Design review of the part built by this model. Coordinates are the model's own, in mm. Face numbers are marked on the shaded views. A direction names the side the tool comes from. Give positions to 0.01 mm unless a question says otherwise; leave off trailing zeros. Write each loop counter-clockwise with the first axis right and the second up, starting at its lowest first coordinate (ties: lowest second). Pieces come first, ordered by that corner, then holes. Notation, with made-up numbers: (-30, 62) -> (14, 62) arc R15 cw to (14, 80) -> close; hole circle Ø1 at (2.25, 27). An arc over 180 degrees is marked (long way). Return JSON: item names as keys, results as strings. Group by question number.
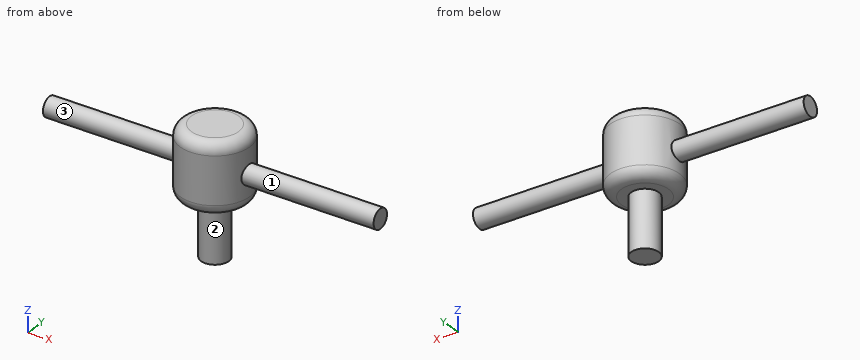
from build123d import *

# Parameters (mm, degrees)
F0_R     = 15.875
F1_DEPTH = 31.75
F2_R     = 4.445
F3_DEPTH = 76.2
F4_R     = 4.445
F5_DEPTH = 76.2
F6_R     = 6.35
F7_DEPTH = 25.908
F8_R     = 5.08


with BuildPart() as f1:
    # F0 (on Top) → F1 (new body)
    with BuildSketch(Plane.XY):
        Circle(F0_R)
    extrude(amount=F1_DEPTH)

    # F2 (on Right) → F3 (join)
    with BuildSketch(Plane.YZ):
        with Locations((0, 14.891451)):
            Circle(F2_R)
    extrude(amount=F3_DEPTH)

    # F4 (on Right) → F5 (join)
    with BuildSketch(Plane.YZ):
        with Locations((0, 14.891451)):
            Circle(F4_R)
    extrude(amount=-F5_DEPTH)

    # F6 (on face) → F7 (join)
    with BuildSketch(Plane(origin=(0, 0, 0), x_dir=(1, 0, 0), z_dir=(0, 0, -1))):
        Circle(F6_R)
    extrude(amount=F7_DEPTH)

    # F8
    f8_edges = [f1.edges().sort_by_distance(p)[0] for p in [
        (-15.875, 0, 31.75),
        (-15.875, 0, 0),
    ]]
    fillet(f8_edges, radius=F8_R)


solid = f1.part
Q1. Insertion check: pin 1 (12 mm diameter, centred on x = 28, z = 6, fed in from +Y); pin 2 (4 mm diameter, centred on y = 11, z = 6, fed in from -X); pin 3 (12 mm diameter, centred on x = -19.5, y = 8, fed in from -Z). Each pin has a flat end and moves straight along its axis. Give the tip position at first contact, or say it passes through.
Q2. Take a section at B-B, the plane x = 0. Give the boundary of the cut face in (y, z) (3 decimals), plus the area to 3 significant figures.
Q3. For L1, parallel to X at y = 4.5, z = 23.5; L2, parallel to Z at x = 62, y = 0.5; L3, parallel to X at y = 8, z = 8.5, list the stretches that pass through material, from the lowest coordinate up. Write a range as from..to.
Q4. Tool access review of the marked faces 1, 2 and 3: name each direction out of +Z, -Z, +X, -X, +Y, -Y from which nothing blocks a thin tool from reaching the whole face with its end or side.
Q5. Take a section at C-C, the plane z = 18. Give the boundary of the cut face in (x, y) (3 decimals), plus the area to 3 significant figures.
Q6. Take a section at A-A, the plane y = 0. Give the boundary of the cut face in (x, z) (3 decimals), plus the area to 3 significant figures.
Q7. Take a section at D-D, the plane z = 6.5. Give the boundary of the cut face in (x, y) (3 decimals), plus the area to 3 significant figures.
Final values:
{
 "1": {"pin 1": "stops at y = 3.38", "pin 2": "stops at x = -13.08", "pin 3": "stops at z = 2.35"},
 "2": {"outline": "(-15.875, 5.08) arc R5.08 ccw to (-10.795, 0) -> (-6.35, 0) -> (-6.35, -25.908) -> (6.35, -25.908) -> (6.35, 0) -> (10.795, 0) arc R5.08 ccw to (15.875, 5.08) -> (15.875, 26.67) arc R5.08 ccw to (10.795, 31.75) -> (-10.795, 31.75) arc R5.08 ccw to (-15.875, 26.67) -> close", "area": "1,310 mm²"},
 "3": {"L1": "x = -15.22..15.22", "L2": "z = 10.47..19.31", "L3": "x = -13.71..13.71"},
 "4": {"face 1": "+X", "face 2": "-Z", "face 3": "-X"},
 "5": {"outline": "(-76.2, -3.177) -> (-15.554, -3.177) arc R15.875 ccw to (15.554, -3.177) -> (76.2, -3.177) -> (76.2, 3.177) -> (15.554, 3.177) arc R15.875 ccw to (-15.554, 3.177) -> (-76.2, 3.177) -> close", "area": "1,560 mm²"},
 "6": {"outline": "(-76.2, 10.446) -> (-15.875, 10.446) -> (-15.875, 5.08) arc R5.08 ccw to (-10.795, 0) -> (-6.35, 0) -> (-6.35, -25.908) -> (6.35, -25.908) -> (6.35, 0) -> (10.795, 0) arc R5.08 ccw to (15.875, 5.08) -> (15.875, 10.446) -> (76.2, 10.446) -> (76.2, 19.336) -> (15.875, 19.336) -> (15.875, 26.67) arc R5.08 ccw to (10.795, 31.75) -> (-10.795, 31.75) arc R5.08 ccw to (-15.875, 26.67) -> (-15.875, 19.336) -> (-76.2, 19.336) -> close", "area": "2,390 mm²"},
 "7": {"outline": "circle Ø31.75 at (0, 0)", "area": "792 mm²"}
}
